Part model, mm, in its own coordinate system. Face numbers are marked on the shaded views. A direction names the side the tool comes from. Round coordinates to 2 decimals unless told otherwise and drop trailing zeros. Write each loop counter-clockwise with the first axis right and the second up, starting at its lowest first coordinate (ties: lowest second). Pieces come first, ordered by that corner, then holes.
```python
from build123d import *

# Parameters (mm, degrees)
EXTRUDE_1_DEPTH     = 8
SKETCH_2_R          = 4
CUT_EXTRUDE_1_DEPTH = 142.73566947
SKETCH_3_W          = 75
SKETCH_3_H          = 8
EXTRUDE_2_DEPTH     = 80
SKETCH_5_R          = 4
CUT_EXTRUDE_2_DEPTH = 147.523035732
RIB_1_REACH         = 156.091
SKETCH_6_WALL_W     = 393.151638598
SKETCH_6_WALL_H     = 8
FILLET_2_R          = 10
EXTRUDE_START       = 3
SKETCH_7_R          = 8
SKETCH_7_R_2        = 4
EXTRUDE_3_DEPTH     = 3
FILLET_3_R          = 1
FILLET_4_R          = 8


with BuildPart() as part:
    # Эскиз1 → Бобышка-Вытянуть1 (new body)
    with BuildSketch(Plane.XY):
        Polygon((0, 0), (75, 0), (75, 30), (55, 120), (0, 120), align=None)
    extrude(amount=EXTRUDE_1_DEPTH)

    # Эскиз2 → Вырез-Вытянуть1 (cut, through all)
    with BuildSketch(Plane.XY.offset(8)):
        with Locations((45, 110)):
            Circle(SKETCH_2_R)
        with Locations((0, 10)):
            Circle(SKETCH_2_R)
        with Locations((65, 10)):
            Circle(SKETCH_2_R)
    extrude(amount=-CUT_EXTRUDE_1_DEPTH, mode=Mode.SUBTRACT)

    # Эскиз3 → Бобышка-Вытянуть2 (add)
    with BuildSketch(Plane.XY.offset(8)):
        with Locations((37.5, 26)):
            Rectangle(SKETCH_3_W, SKETCH_3_H)
    extrude(amount=EXTRUDE_2_DEPTH)

    # Эскиз5 → Вырез-Вытянуть2 (cut, through all)
    with BuildSketch(Plane(origin=(0, 30, 0), x_dir=(1, 0, 0), z_dir=(0, 1, 0))):
        with Locations(Location((50, -30.5, 0), (0, 0, 270))):
            Circle(SKETCH_5_R)
        with Locations(Location((50, -65.5, 0), (0, 0, 270))):
            Circle(SKETCH_5_R)
    extrude(amount=-CUT_EXTRUDE_2_DEPTH, mode=Mode.SUBTRACT)

    # Эскиз6 wall → Ребро1 (add, up to next)
    with BuildSketch(Plane(origin=(35, 11, 48), x_dir=(0, -0.265156483021, -0.964205392804), z_dir=(0, 0.964205392804, -0.265156483021)), mode=Mode.PRIVATE) as rib_1_sk1:
        Rectangle(SKETCH_6_WALL_W, SKETCH_6_WALL_H)
    rib_1_tool1 = extrude(rib_1_sk1.sketch, amount=RIB_1_REACH, mode=Mode.PRIVATE) - part.part
    add(rib_1_tool1.solids().sort_by_distance((35, 11, 48))[0])

    # Скругление2
    fillet_2_edges = [part.edges().sort_by_distance(p)[0] for p in [
        (55, 120, 4),
        (75, 0, 4),
        (75, 26, 88),
    ]]
    fillet(fillet_2_edges, radius=FILLET_2_R)

    # Зеркальное отражение1: part across plane


with BuildPart() as part_1:
    add(part.part)
    add(part.part.mirror(Plane(origin=(0, 120, 8), x_dir=(0, 0, 1), z_dir=(1, 0, 0))))

    # Эскиз7 → Бобышка-Вытянуть3 (add)
    # profile 1 of 2: a face of its own
    with BuildSketch(Plane.XY.offset(8).offset(EXTRUDE_START)):
        with Locations((-45, 110)):
            Circle(SKETCH_7_R)
        with Locations(Location((-45, 110, 0), (0, 0, 180))):
            Circle(SKETCH_7_R_2, mode=Mode.SUBTRACT)
    # profile 2 of 2: a face of its own
    with BuildSketch(Plane.XY.offset(8).offset(EXTRUDE_START)):
        with Locations((45, 110)):
            Circle(SKETCH_7_R)
        with Locations((45, 110)):
            Circle(SKETCH_7_R_2, mode=Mode.SUBTRACT)
    extrude(amount=-EXTRUDE_3_DEPTH)

    # Скругление3
    fillet_3_edges = [part_1.edges().sort_by_distance(p)[0] for p in [
        (-53, 110, 8),
        (37, 110, 8),
    ]]
    fillet(fillet_3_edges, radius=FILLET_3_R)

    # Скругление4
    fillet_4_edges = [part_1.edges().sort_by_distance(p)[0] for p in [
        (-39, 11, 8),
        (-31, 11, 8),
        (31, 11, 8),
        (39, 11, 8),
    ]]
    fillet(fillet_4_edges, radius=FILLET_4_R)


solid = part_1.part
```
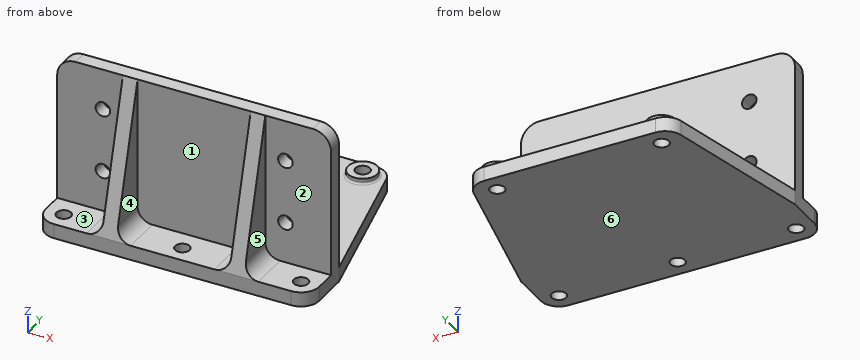
Q1. Wall check: L1, parallel to Z at x = -50, y = 28; L2, parallel to X at y = 24, z = 65; L3, parallel to X at y = 20, z = 20. Give the ranges that are in metal, low to high.
Values follow:
L1: z = 0 to 26.5, 34.5 to 61.5, 69.5 to 88
L2: x = -75 to -53.97, -46.03 to 46.03, 53.97 to 75
L3: x = -39 to -31, 31 to 39
Q2. Mould opens along X. For the marked faces 4, 5 and 6 say: +X half, -X half, draft (parallel to the pull), parting line (faces both ways), or undercut.
Values follow:
face 4: undercut
face 5: +X half
face 6: draft
Q3. Cut at A-A on x = 0. Write the cut outline in (y, z), plus the area to 3 significant figures.
Values follow:
outline: (0, 0) - (6, 0) - (6, 8) - (0, 8) - close; (14, 0) - (120, 0) - (120, 8) - (30, 8) - (30, 88) - (22, 88) - (22, 8) - (14, 8) - close
area: 1,540 mm2
Q4. Which spindle directions (+Z, -Z, +X, -X, +Y, -Y) get a long thin tool onto all of the face, cutting with end or side? Do the marked faces 1, 2 and 3. Say none if no direction does.
Values follow:
face 1: +Z, -Y
face 2: +Z, +X, -Y
face 3: +Z, -X, -Y
Q5. Drop flat-ended pins along their axis: pin 1 (16 mm diameter, centred on y = 7.5, z = 56, fed in from -X); pin 2 (5 mm diameter, centred on x = 37, z = 72.5, fed in from +Y); pin 3 (5 mm diameter, centred on x = -34.5, z = 21.5, fed in from -Y) (3 decimals). Give the stop position or say it passes through.
Values follow:
pin 1: stops at x = -39
pin 2: stops at y = 30
pin 3: stops at y = 3.025
Q6. Cut at D-D on x = -33. Write the cut outline in (y, z), plus the area to 3 significant figures.
Values follow:
outline: (0, 0) - (120, 0) - (120, 8) - (30, 8) - (30, 88) - (22, 88) - (0, 8) - close
area: 2,480 mm2
Q7. Cut at C-C on z = 22. Write the cut outline in (x, y), plus the area to 3 significant figures.
Values follow:
outline: (-75, 22) - (-39, 22) - (-39, 3.85) - (-31, 3.85) - (-31, 22) - (31, 22) - (31, 3.85) - (39, 3.85) - (39, 22) - (75, 22) - (75, 30) - (-75, 30) - close
area: 1,490 mm2
Q8. Cut at B-B on z = 65.5. Write the cut outline in (x, y), plus the area to 3 significant figures.
Values follow:
outline: (-75, 22) - (-54, 22) - (-54, 30) - (-75, 30) - close; (-46, 22) - (-39, 22) - (-39, 15.81) - (-31, 15.81) - (-31, 22) - (31, 22) - (31, 15.81) - (39, 15.81) - (39, 22) - (46, 22) - (46, 30) - (-46, 30) - close; (54, 22) - (75, 22) - (75, 30) - (54, 30) - close
area: 1,170 mm2
